from build123d import *

# Parameters (mm, degrees)
SKETCH1_R           = 60
SKETCH1_R_2         = 43.5
EXTRUSION1_DEPTH    = 60
EXTRUSION3_START    = -60
EXTRUSION3_DEPTH    = 60
BOSS_EXTRUDE1_DEPTH = 60


with BuildPart() as part:
    # Sketch1 → Extrusion1 (new body)
    with BuildSketch(Plane.XY):
        Circle(SKETCH1_R)
        Circle(SKETCH1_R_2, mode=Mode.SUBTRACT)
    extrude(amount=EXTRUSION1_DEPTH)

    # Sketch3 → Extrusion3 (cut)
    with BuildSketch(Plane.XY.offset(60).offset(EXTRUSION3_START)):
        with BuildLine():
            Line((-0.5, 48.5), (-0.5, 43.497126342))
            ThreePointArc((-0.5, 43.497126342), (0, 43.5), (0.5, 43.497126342))
            Line((0.5, 43.497126342), (0.5, 48.5))
            Line((0.5, 48.5), (-0.5, 48.5))
        make_face()
    extrude(amount=EXTRUSION3_DEPTH, mode=Mode.SUBTRACT)

    # Sketch4 → Boss-Extrude1 (add, through all)
    with BuildSketch(Plane.XY.offset(60)):
        with BuildLine():
            Line((41.352486375, 43.473806719), (48.436814511, 50.558134855))
            Line((48.436814511, 50.558134855), (50.558134855, 48.436814511))
            Line((50.558134855, 48.436814511), (43.473806719, 41.352486375))
            ThreePointArc((43.473806719, 41.352486375), (42.426406871, 42.426406871), (41.352486375, 43.473806719))
        make_face()
        with BuildLine():
            Line((1.5, 59.981247069), (1.5, 70))
            Line((1.5, 70), (-1.5, 70))
            Line((-1.5, 70), (-1.5, 59.981247069))
            ThreePointArc((-1.5, 59.981247069), (0, 60), (1.5, 59.981247069))
        make_face()
        with BuildLine():
            Line((59.981247069, 1.5), (70, 1.5))
            Line((70, 1.5), (70, -1.5))
            Line((70, -1.5), (59.981247069, -1.5))
            ThreePointArc((59.981247069, -1.5), (60, 0), (59.981247069, 1.5))
        make_face()
        with BuildLine():
            Line((43.473806719, -41.352486375), (50.558134855, -48.436814511))
            Line((50.558134855, -48.436814511), (48.436814511, -50.558134855))
            Line((48.436814511, -50.558134855), (41.352486375, -43.473806719))
            ThreePointArc((41.352486375, -43.473806719), (42.426406871, -42.426406871), (43.473806719, -41.352486375))
        make_face()
        with BuildLine():
            Line((1.5, -59.981247069), (1.5, -70))
            Line((1.5, -70), (-1.5, -70))
            Line((-1.5, -70), (-1.5, -59.981247069))
            ThreePointArc((-1.5, -59.981247069), (0, -60), (1.5, -59.981247069))
        make_face()
        with BuildLine():
            Line((-41.352486375, -43.473806719), (-48.436814511, -50.558134855))
            Line((-48.436814511, -50.558134855), (-50.558134855, -48.436814511))
            Line((-50.558134855, -48.436814511), (-43.473806719, -41.352486375))
            ThreePointArc((-43.473806719, -41.352486375), (-42.426406871, -42.426406871), (-41.352486375, -43.473806719))
        make_face()
        with BuildLine():
            Line((-59.981247069, -1.5), (-70, -1.5))
            Line((-70, -1.5), (-70, 1.5))
            Line((-70, 1.5), (-59.981247069, 1.5))
            ThreePointArc((-59.981247069, 1.5), (-60, 0), (-59.981247069, -1.5))
        make_face()
        with BuildLine():
            Line((-43.473806719, 41.352486375), (-50.558134855, 48.436814511))
            Line((-50.558134855, 48.436814511), (-48.436814511, 50.558134855))
            Line((-48.436814511, 50.558134855), (-41.352486375, 43.473806719))
            ThreePointArc((-41.352486375, 43.473806719), (-42.426406871, 42.426406871), (-43.473806719, 41.352486375))
        make_face()
    extrude(amount=-BOSS_EXTRUDE1_DEPTH)


solid = part.part
For this review, take the finished solid that the model builds, in its own axes (mm). A direction names the side the tool comes from. Round coordinates to 2 decimals unless told otherwise and drop trailing zeros. Loops run counter-clockwise (first coordinate to the right, second up) from the corner with the lowest first, then second, coordinate; pieces in that order, holes last. Notation, with made-up numbers: (-36, 38.25) - (-29, 38.25) arc R11 cw to (-29, 51.25) - close; hole circle Ø7 at (76.25, 48). An arc over 180 degrees is marked (long way). Answer as CSV lines item,"result".
(1) Mouldability with a two-part tool opening along Y and no side actions: class faces 1 (the face through (22.68, -55.55, 29.58)), 2 (the face through (1.5, -65, 30)), 3 (the face through (46.97, -44.85, 30.42)) as +Y half, -Y half, draft (parallel to the pull), parting line (faces both ways), or undercut.
Checked values:
face 1,"-Y half"
face 2,"draft"
face 3,"undercut"
(2) Consider section D-D on x = -53.5. Give the boundary of the cut face in (y, z).
Checked values:
outline,"(-27.16, 0) - (27.16, 0) - (27.16, 60) - (-27.16, 60) - close"
(3) Consider section C-C on y = 56. Give the boundary of the cut face in (x, z).
Checked values:
outline,"(-21.54, 0) - (21.54, 0) - (21.54, 60) - (-21.54, 60) - close"
(4) Insertion check: P1, Ø1.5, axis at y = -44, z = 26.5, coming from the -X side; P2, Ø6, axis at y = -21, z = 44, coming from the +X side; P3, Ø12, axis at x = 8.5, y = -47.5, coming from the -Z side; P4, Ø4, axis at y = -40.5, z = 51.5, coming from the +X side. Each pin has a flat end and moves straight along its axis. Give the tip position at first contact, or say it passes through.
Checked values:
P1,"stops at x = -46.87"
P2,"stops at x = 57.24"
P3,"stops at z = 0"
P4,"stops at x = 46.02"
(5) Wall thickness on line 1 (X direction, y = 0, z = 33); line 2 (Y direction, x = 0, z = 32); line 3 (X direction, y = -48, z = 20): over which ranges is each line inside the solid? List them lowest first.
Checked values:
line 1,"x = -70 to -43.5, 43.5 to 70"
line 2,"y = -70 to -43.5, 48.5 to 70"
line 3,"x = -50.12 to -45.88, -36 to 36, 45.88 to 50.12"
(6) Consider section A-A on x = -39. Give the boundary of the cut face in (y, z).
Checked values:
outline,"(-45.6, 0) - (-19.27, 0) - (-19.27, 60) - (-45.6, 60) - close; (19.27, 0) - (45.6, 0) - (45.6, 60) - (19.27, 60) - close"
(7) Tool access review of faces 4 (the face through (65, -1.5, 30)), 5 (the face through (23.246, 55.314, 29.58)), 6 (the face through (-55.55, -22.68, 29.58)), 7 (the face through (-65, -1.5, 30)): name each direction out of +Z, -Z, +X, -X, +Y, -Y from which nothing blocks a thin tool from reaching the whole face with its end or side.
Checked values:
face 4,"+Z, -Z, +X, -Y"
face 5,"+Z, -Z, +Y"
face 6,"+Z, -Z, -X"
face 7,"+Z, -Z, -X, -Y"
(8) Consider section B-B on y = -14. Give the boundary of the cut face in (x, z).
Checked values:
outline,"(-58.34, 0) - (-41.19, 0) - (-41.19, 60) - (-58.34, 60) - close; (41.19, 0) - (58.34, 0) - (58.34, 60) - (41.19, 60) - close"
